from build123d import *

# Parameters (mm, degrees)
SKETCH_1_W          = 47.5
SKETCH_1_H          = 90
SKETCH_1_R          = 1.5
EXTRUDE_1_DEPTH     = 4
SKETCH_2_R          = 1.5
SKETCH_2_W          = 35.5
SKETCH_2_H          = 60
SKETCH_2_W_2        = 8.75
SKETCH_2_H_2        = 24
SKETCH_2_W_3        = 20
SKETCH_2_H_3        = 17.7
CUT_EXTRUDE_2_DEPTH = 94.166853011
FILLET_1_R          = 2


with BuildPart() as part:
    # 草图1 → 凸台-拉伸1 (new body)
    with BuildSketch(Plane(origin=(0, 0, 0), x_dir=(1, 0, 0), z_dir=(0, 1, 0))):
        with Locations((0, 45)):
            Rectangle(SKETCH_1_W, SKETCH_1_H)
        with Locations(Location((-10, 27, 0), (0, 0, 270))):
            Circle(SKETCH_1_R, mode=Mode.SUBTRACT)
        with Locations(Location((0, 3.3, 0), (0, 0, 270))):
            Circle(SKETCH_1_R, mode=Mode.SUBTRACT)
        with Locations(Location((10, 27, 0), (0, 0, 90))):
            Circle(SKETCH_1_R, mode=Mode.SUBTRACT)
    extrude(amount=EXTRUDE_1_DEPTH)

    # 草图2 → 切除-拉伸2 (cut, through all)
    with BuildSketch(Plane(origin=(0, 0, 0), x_dir=(1, 0, 0), z_dir=(0, 1, 0))):
        with Locations(Location((-20.75, 87, 0), (0, 0, 270))):
            Circle(SKETCH_2_R)
        with Locations(Location((20.75, 87, 0), (0, 0, 90))):
            Circle(SKETCH_2_R)
        with Locations(Location((-20.75, 27, 0), (0, 0, 270))):
            Circle(SKETCH_2_R)
        with Locations(Location((20.75, 27, 0), (0, 0, 90))):
            Circle(SKETCH_2_R)
        with Locations((0, 60)):
            Rectangle(SKETCH_2_W, SKETCH_2_H)
        with Locations((-19.375, 12)):
            Rectangle(SKETCH_2_W_2, SKETCH_2_H_2)
        with Locations((19.375, 12)):
            Rectangle(SKETCH_2_W_2, SKETCH_2_H_2)
        with Locations((0, 15.15)):
            Rectangle(SKETCH_2_W_3, SKETCH_2_H_3)
    extrude(amount=CUT_EXTRUDE_2_DEPTH, mode=Mode.SUBTRACT)

    # 圆角1
    fillet_1_edges = [part.edges().sort_by_distance(p)[0] for p in [
        (-23.75, 2, -24),
        (-15, 2, 0),
        (-15, 2, -24),
        (-10, 2, -24),
        (-10, 2, -6.3),
        (10, 2, -6.3),
        (10, 2, -24),
        (23.75, 2, -24),
        (15, 2, -24),
        (15, 2, 0),
        (-17.75, 2, -90),
        (-17.75, 2, -30),
        (17.75, 2, -30),
        (17.75, 2, -90),
        (-23.75, 2, -90),
        (23.75, 2, -90),
    ]]
    fillet(fillet_1_edges, radius=FILLET_1_R)


solid = part.part
Geometry check sheet. Reference: the model listing, model coordinates, mm. A direction names the side the tool comes from. Coordinates: 2 decimals unless noted, no trailing zeros. Order: outer loops, then holes, each group sorted by start corner. A loop starts at its lowest first (then second) coordinate and runs counter-clockwise, first axis right, second up. Notation, with made-up numbers: M -36.75,-21.5 L -8.75,-21.5 A13 cw -8.75,-15.5 Z; hole C 10.25,89 d3. An arc over 180 degrees is marked long. Use CSV: the item, a comma, the result in double quotes.
Item 1: Tool access check on faces 4 (the flat face through (-23.75, 2, -57)), 5 (the flat face through (15, 2, -12)), 6 (the cylindrical face through (17.15, 2.03, -30.57)), 7 (the flat face through (-19, 2, -24)), 8 (the cylindrical face through (-9.4, 2.03, -23.43)). Record the directions out of +Z, -Z, +X, -X, +Y, -Y that give a thin tool (end or side, any length) a straight path to the whole face; none if there is none.
Returned:
face 4,"+Z, -Z, -X, +Y, -Y"
face 5,"+Z, +X, +Y, -Y"
face 6,"-Z, +Y, -Y"
face 7,"+Z, -X, +Y, -Y"
face 8,"+Y, -Y"
Item 2: Cross-section at C-C on z = -27. Record the cut outline in (x, y).
Returned:
outline,"M -23.75,0 L -22.25,0 L -22.25,4 L -23.75,4 Z; M -19.25,0 L -11.5,0 L -11.5,4 L -19.25,4 Z; M -8.5,0 L 8.5,0 L 8.5,4 L -8.5,4 Z; M 11.5,0 L 19.25,0 L 19.25,4 L 11.5,4 Z; M 22.25,0 L 23.75,0 L 23.75,4 L 22.25,4 Z"
Item 3: Thickness scan on line 1 along Z through (x, y) = (20.75, 1.1); line 2 along X through (y, z) = (1.3, -87); line 3 along X through (y, z) = (2.6, -27). Record the ranges inside material, lowest first.
Returned:
line 1,"z = -90 to -88.5, -85.5 to -28.5, -25.5 to -24"
line 2,"x = -23.75 to -22.25, -19.25 to -17.75, 17.75 to 19.25, 22.25 to 23.75"
line 3,"x = -23.75 to -22.25, -19.25 to -11.5, -8.5 to 8.5, 11.5 to 19.25, 22.25 to 23.75"
Item 4: Gauge pin test, flat ends, axial feed: pin 1 Ø2 at (y, z) = (3, -12.5) entering from -X; pin 2 Ø2 at (x, y) = (6, 2) entering from -Z; pin 3 Ø1.2 at (y, z) = (1.5, -13) entering from +X. Record the tip position at first contact, or that the pin passes through.
Returned:
pin 1,"stops at x = -15"
pin 2,"stops at z = -30"
pin 3,"stops at x = 15"
Item 5: Cross-section at D-D on x = 20.75. Record the cut outline in (y, z), then the cut area to 3 significant figures.
Returned:
outline,"M 0,-90 L 4,-90 L 4,-88.5 L 0,-88.5 Z; M 0,-85.5 L 4,-85.5 L 4,-28.5 L 0,-28.5 Z; M 0,-25.5 L 4,-25.5 L 4,-24 L 0,-24 Z"
area,"240 mm2"
Item 6: Cross-section at A-A on z = -42. Record the cut outline in (x, y), then the cut area to 3 significant figures.
Returned:
outline,"M -23.75,0 L -17.75,0 L -17.75,4 L -23.75,4 Z; M 17.75,0 L 23.75,0 L 23.75,4 L 17.75,4 Z"
area,"48.0 mm2"
Item 7: Cross-section at B-B on x = -3. Record the cut outline in (y, z).
Returned:
outline,"M 0,-30 L 4,-30 L 4,-24 L 0,-24 Z; M 0,-6.3 L 4,-6.3 L 4,0 L 0,0 Z"
Item 8: Mould release check, pull along X, two halves, no side actions. Record for faces 1 (the cylindrical face through (14.43, 2.03, -0.6)), 2 (the flat face through (-10, 2, -15)), 3 (the cylindrical face through (-23.18, 2.03, -89.4)): pulls with the +X half, pulls with the -X half, needs draft (parallel to the pull), parting line crosses it, or undercut.
Returned:
face 1,"pulls with the +X half"
face 2,"undercut"
face 3,"pulls with the -X half"
